Can you work these out from the model? Positions are in its coordinate system, mm. Give positions to 0.01 mm unless a question says otherwise; leave off trailing zeros. Order: outer loops, then holes, each group sorted by start corner. A loop starts at its lowest first (then second) coordinate and runs counter-clockwise, first axis right, second up. Notation, with made-up numbers: M 44,13 L 74,13 A9 ccw 74,22 Z; hole C 27.5,26.25 d7. An arc over 180 degrees is marked long. Use one line per item in the form item = value. Start each with the question number.
1. I want a section at C-C, the plane y = -4.5. List the corners of the cut face in (x, z) for me, and give its area (3 significant figures).
2. I want a section at B-B, the plane y = 0. List the corners of the cut face in (x, z) for me, and give its area (3 significant figures).
3. I need wall thicknesses on L1, parallel to X at y = -6.5, z = 1.7; L2, parallel to X at y = 8, z = 2.3; L3, parallel to X at y = -7.75, z = 1.8. Which ranges of each line are inside material? Lowest first, please.
4. I want a section at A-A, the plane x = 0. List the corners of the cut face in (y, z) for me, and give its area (3 significant figures).
5. Will these pins go through, and if not, where does the flat tip stop? P1, Ø1, axis at x = -9.5, z = 1, coming from the -Y side; P2, Ø1.5, axis at y = 7.5, z = 1, coming from the +X side; P3, Ø1.5, axis at x = 11, z = 2, coming from the -Y side.
6. I want a section at D-D, the plane z = 2.2. Count the separate pieces of the cut face and the enclosed holes in it, and give its area (3 significant figures).
Autodesk Inventor part; units mm, degrees
ref_plane "YZ Plane" through (0, 0, 0) normal (1, 0, 0) x (0, 1, 0)
ref_plane "XZ Plane" through (0, 0, 0) normal (0, 1, 0) x (-1, 0, 0)
ref_plane "XY Plane" through (0, 0, 0) normal (0, 0, 1) x (1, 0, 0)
sketch "Boceto1" plane through (0, 0, 0) normal (0, 0, 1) x (1, 0, 0)
  circle A0 centre (0, 0) radius 15
  circle A1 centre (0, 0) radius 2.8
  line L0 (-1.852, 2.1) -> (1.852, 2.1)
  line L1 (-1.852, -2.1) -> (1.852, -2.1)
  dimension "d0" = 30
  dimension "d1" = 5.6
  dimension "d2" = 2.1
  dimension "d3" = 2.1
extrude "Extrusión1" add sketch "Boceto1" along normal blind 3 contours A0 | L0 A1 | A1 L1
sketch "Boceto2" plane through (0, 0, 3) normal (0, 0, 1) x (1, 0, 0)
  line L0 (-0.875, 13) -> (0.875, 13)
  line L1 (0.875, 13) -> (0.875, 9.5)
  line L2 (0.875, 9.5) -> (-0.875, 9.5)
  line L3 (-0.875, 9.5) -> (-0.875, 13)
  point P0 (0, 0)
  point P1 (0, 13)
  dimension "d6" = 3.5
  dimension "d7" = 1.75
  dimension "d8" = 9.5
extrude "Extrusión2" cut sketch "Boceto2" against normal through all
pattern_circular "Patrón circular1" count 20 over 360 about axis through (0, 0, -10) along (0, 0, 1) of "Extrusión2"
properties part number "Disco_encoder"
Check result:
q1.outline = M -14.31,0 L -12.21,0 L -12.21,3 L -14.31,3 Z; M -11.02,0 L 11.02,0 L 11.02,3 L -11.02,3 Z; M 12.21,0 L 14.31,0 L 14.31,3 L 12.21,3 Z
q1.area = 78.7 mm2
q2.outline = M -15,0 L -13,0 L -13,3 L -15,3 Z; M -9.5,0 L -2.8,0 L -2.8,3 L -9.5,3 Z; M 2.8,0 L 9.5,0 L 9.5,3 L 2.8,3 Z; M 13,0 L 15,0 L 15,3 L 13,3 Z
q2.area = 52.2 mm2
q3.L1 = -13.52 to -10.44, -7.46 to 7.46, 10.44 to 13.52
q3.L2 = -12.69 to -10.26, -9.52 to -6.89, -5.15 to 5.15, 6.89 to 9.52, 10.26 to 12.69
q3.L3 = -12.84 to -10.44, -9.18 to -6.71, -5.5 to 5.5, 6.71 to 9.18, 10.44 to 12.84
q4.outline = M -15,0 L -13,0 L -13,3 L -15,3 Z; M -9.5,0 L -2.1,0 L -2.1,3 L -9.5,3 Z; M 2.1,0 L 9.5,0 L 9.5,3 L 2.1,3 Z; M 13,0 L 15,0 L 15,3 L 13,3 Z
q4.area = 56.4 mm2
q5.P1 = -12
q5.P2 = 13.4
q5.P3 = -10.95
q6.separate_pieces = 1
q6.enclosed_holes = 21
q6.area = 563 mm2
